The model under review builds one solid part; all positions refer to its coordinate system, in mm. A direction names the side the tool comes from. Give positions to 0.01 mm unless a question says otherwise; leave off trailing zeros. Order: outer loops, then holes, each group sorted by start corner. A loop starts at its lowest first (then second) coordinate and runs counter-clockwise, first axis right, second up.
```python
from build123d import *

# Parameters (mm, degrees)
SKETCH_1_W          = 60
SKETCH_1_H          = 50
EXTRUDE_1_DEPTH     = 2
SKETCH_2_W          = 10
SKETCH_2_H          = 2
EXTRUDE_2_DEPTH     = 60
SKETCH_3_R          = 1.6
CUT_EXTRUDE_1_DEPTH = 51
FILLET_1_R          = 2


with BuildPart() as part:
    # 草图1 → 凸台-拉伸1 (new body)
    with BuildSketch(Plane.XY):
        with Locations((-50.970873786, -63.980582524)):
            Rectangle(SKETCH_1_W, SKETCH_1_H)
        Polygon((-77.970873786, -45.804555709), (-77.970873786, -82.156609339), (-66.817402786, -63.980582524), align=None, mode=Mode.SUBTRACT)
        Polygon((-75.624344787, -85.980582524), (-53.317402786, -85.980582524), (-64.470873786, -67.804555709), align=None, mode=Mode.SUBTRACT)
        Polygon((-23.970873786, -45.9315118), (-23.970873786, -82.156609339), (-34.838542531, -64.446334348), align=None, mode=Mode.SUBTRACT)
        Polygon((-75.596017187, -41.980582524), (-53.317402786, -41.980582524), (-64.219831603, -59.747503559), align=None, mode=Mode.SUBTRACT)
        Polygon((-50.970873786, -45.804555709), (-39.503543881, -64.492056295), (-49.871707725, -82.155891862), (-61.82340345, -63.490159606), align=None, mode=Mode.SUBTRACT)
        Polygon((-26.289955727, -41.980582524), (-37.209130522, -60.583153918), (-48.624344787, -41.980582524), align=None, mode=Mode.SUBTRACT)
        Polygon((-37.13295589, -68.355236725), (-26.317402786, -85.980582524), (-47.478527346, -85.980582524), align=None, mode=Mode.SUBTRACT)
    extrude(amount=EXTRUDE_1_DEPTH)

    # 草图2 → 凸台-拉伸2 (add)
    with BuildSketch(Plane(origin=(-20.970873786, 0, 0), x_dir=(0, 0, -1), z_dir=(1, 0, 0))):
        with Locations((-7, -87.980582524)):
            Rectangle(SKETCH_2_W, SKETCH_2_H)
        with Locations((-7, -39.980582524)):
            Rectangle(SKETCH_2_W, SKETCH_2_H)
    extrude(amount=-EXTRUDE_2_DEPTH)

    # 草图3 → 切除-拉伸1 (cut, through all)
    with BuildSketch(Plane(origin=(0, -38.980582524, 0), x_dir=(1, 0, 0), z_dir=(0, 1, 0))):
        with Locations((-75.970873786, -7)):
            Circle(SKETCH_3_R)
        with Locations((-65.970873786, -7)):
            Circle(SKETCH_3_R)
        with Locations((-35.970873786, -7)):
            Circle(SKETCH_3_R)
        with Locations((-25.970873786, -7)):
            Circle(SKETCH_3_R)
    extrude(amount=-CUT_EXTRUDE_1_DEPTH, mode=Mode.SUBTRACT)

    # 圆角1
    fillet_1_edges = [part.edges().sort_by_distance(p)[0] for p in [
        (-50.970873786, -45.804555709, 1),
        (-61.82340345, -63.490159606, 1),
        (-49.871707725, -82.155891862, 1),
        (-39.503543881, -64.492056295, 1),
        (-66.817402786, -63.980582524, 1),
        (-77.970873786, -45.804555709, 1),
        (-77.970873786, -82.156609339, 1),
        (-75.596017187, -41.980582524, 1),
        (-64.219831603, -59.747503559, 1),
        (-53.317402786, -41.980582524, 1),
        (-26.289955727, -41.980582524, 1),
        (-48.624344787, -41.980582524, 1),
        (-37.209130522, -60.583153918, 1),
        (-23.970873786, -45.9315118, 1),
        (-34.838542531, -64.446334348, 1),
        (-23.970873786, -82.156609339, 1),
        (-64.470873786, -67.804555709, 1),
        (-75.624344787, -85.980582524, 1),
        (-53.317402786, -85.980582524, 1),
        (-47.478527346, -85.980582524, 1),
        (-26.317402786, -85.980582524, 1),
        (-37.13295589, -68.355236725, 1),
    ]]
    fillet(fillet_1_edges, radius=FILLET_1_R)


solid = part.part
```
Item 1: Take a section at D-D (y = -60.5). Give the boundary of the cut face in (x, z), and give its area (3 significant figures).
Values found:
outline: (-80.97, 0) - (-77.97, 0) - (-77.97, 2) - (-80.97, 2) - close; (-68.95, 0) - (-59.99, 0) - (-59.99, 2) - (-68.95, 2) - close; (-41.95, 0) - (-32.52, 0) - (-32.52, 2) - (-41.95, 2) - close; (-23.97, 0) - (-20.97, 0) - (-20.97, 2) - (-23.97, 2) - close
area: 48.8 mm2
Item 2: Take a section at C-C (y = -82). Give the boundary of the cut face in (x, z), and give its area (3 significant figures).
Values found:
outline: (-80.97, 0) - (-73.18, 0) - (-73.18, 2) - (-80.97, 2) - close; (-55.76, 0) - (-45.14, 0) - (-45.14, 2) - (-55.76, 2) - close; (-28.76, 0) - (-20.97, 0) - (-20.97, 2) - (-28.76, 2) - close
area: 52.4 mm2
Item 3: Take a section at A-A (z = 11). Give the boundary of the cut face in (x, y), and give its area (3 significant figures).
Values found:
outline: (-80.97, -88.98) - (-20.97, -88.98) - (-20.97, -86.98) - (-80.97, -86.98) - close; (-80.97, -40.98) - (-20.97, -40.98) - (-20.97, -38.98) - (-80.97, -38.98) - close
area: 240 mm2
Item 4: Clearance check with a flat-ended pin moving along its axis: pin 1 Ø2 at (y, z) = (-72.5, 3.5) entering from -X. State where the tip first meets the part, or that it passes through.
Values found:
pin 1: passes through
Item 5: Take a section at B-B (x = -42). Give the boundary of the cut face in (y, z).
Values found:
outline: (-88.98, 0) - (-85.98, 0) - (-85.98, 2) - (-86.98, 2) - (-86.98, 12) - (-88.98, 12) - close; (-76.65, 0) - (-68.75, 0) - (-68.75, 2) - (-76.65, 2) - close; (-60.42, 0) - (-52.78, 0) - (-52.78, 2) - (-60.42, 2) - close; (-41.98, 0) - (-38.98, 0) - (-38.98, 12) - (-40.98, 12) - (-40.98, 2) - (-41.98, 2) - close
Item 6: Draft analysis for pull direction Y (two halves, no side actions). For faces 1 (the flat face through (-37, -85.981, 1)), 2 (the flat face through (-77.971, -64, 1)), 3 (the cylindrical face through (-37.241, -39.967, 7.974)), 4 (the flat face through (-51, -88.981, 6)), state which applies: released by +Y, released by -Y, zero draft, split by the parting line, or undercut.
Values found:
face 1: undercut
face 2: undercut
face 3: zero draft
face 4: released by -Y
Item 7: For line 1 (X direction, y = -87.85, z = 7); line 2 (X direction, y = -85, z = 0.5); line 3 (Y direction, x = -42.5, z = 1.25), list the stretches that pass through material, from the lowest coordinate up.
Values found:
line 1: x = -80.97 to -77.57, -74.37 to -67.57, -64.37 to -37.57, -34.37 to -27.57, -24.37 to -20.97
line 2: x = -80.97 to -73.77, -55.17 to -45.71, -28.17 to -20.97
line 3: y = -88.98 to -85.98, -77.5 to -69.6, -59.61 to -51.96, -41.98 to -38.98
Item 8: For faces 5 (the flat face through (-20.971, -65.7, 1.6)), 6 (the flat face through (-51, -40.981, 7)), 7 (the cylindrical face through (-64.5, -69.63, 1.01)), list the 3-axis set-ups (+Z, -Z, +X, -X, +Y, -Y) from which the entire face can be reached by the end or side of a thin tool; tool diameter is ignored.
Values found:
face 5: +Z, -Z, +X, +Y, -Y
face 6: +Z, +X, -X
face 7: +Z, -Z
